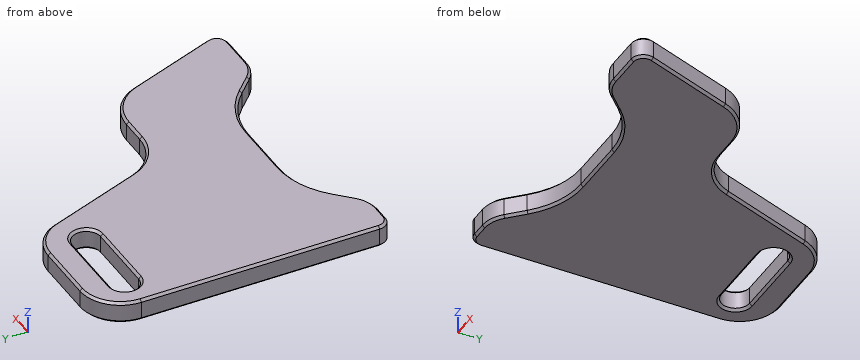
from build123d import *

# Parameters (mm, degrees)
BOSS_EXTRU_1_DEPTH           = 27
ENL_V_MAT_EXTRU_1_DEPTH      = 544.312782602
ENL_V_MAT_EXTRU_1_DEPTH_BACK = 544.312782602
CONG_3_R                     = 60
CONG_4_R                     = 50
CONG_5_R                     = 100
CONG_6_R                     = 15
CONG_7_R                     = 40
ENL_V_MAT_EXTRU_2_DEPTH      = 539.530227365
ENL_V_MAT_EXTRU_2_DEPTH_BACK = 539.530227365
CHANFREIN1_SIZE              = 3


with BuildPart() as part:
    # Esquisse1 → Boss.-Extru.1 (new body)
    with BuildSketch(Plane.XY):
        Polygon((0, 0), (0, 360), (160, 360), (229.154344511, 170), (344.154344511, 170), (406.029284336, 0), align=None)
    extrude(amount=BOSS_EXTRU_1_DEPTH)

    # Esquisse2 → Enlèv. mat.-Extru.1 (cut, two sides: drawn at the far end of the back side and taken through both)
    with BuildSketch(Plane.XY.offset(27).offset(-ENL_V_MAT_EXTRU_1_DEPTH_BACK)):
        Polygon((50, 0), (110, 60), (266.029284336, 60), (326.029284336, 0), align=None)
    extrude(amount=ENL_V_MAT_EXTRU_1_DEPTH + ENL_V_MAT_EXTRU_1_DEPTH_BACK, mode=Mode.SUBTRACT)

    # Congé3
    cong_3_edges = [part.edges().sort_by_distance(p)[0] for p in [
        (229.154344511, 170, 13.5),
        (344.154344511, 170, 13.5),
    ]]
    fillet(cong_3_edges, radius=CONG_3_R)

    # Congé4
    cong_4_edges = [part.edges().sort_by_distance(p)[0] for p in [
        (0, 360, 13.5),
        (160, 360, 13.5),
    ]]
    fillet(cong_4_edges, radius=CONG_4_R)

    # Congé5
    cong_5_edges = [part.edges().sort_by_distance(p)[0] for p in [
        (110, 60, 13.5),
        (266.029284336, 60, 13.5),
    ]]
    fillet(cong_5_edges, radius=CONG_5_R)

    # Congé6
    cong_6_edges = [part.edges().sort_by_distance(p)[0] for p in [
        (0, 0, 13.5),
        (406.029284336, 0, 13.5),
    ]]
    fillet(cong_6_edges, radius=CONG_6_R)

    # Congé7
    cong_7_edges = [part.edges().sort_by_distance(p)[0] for p in [
        (326.029284336, 0, 13.5),
        (50, 0, 13.5),
    ]]
    fillet(cong_7_edges, radius=CONG_7_R)

    # Esquisse3 → Enlèv. mat.-Extru.2 (cut, two sides: drawn at the far end of the back side and taken through both)
    with BuildSketch(Plane.XY.offset(27).offset(-ENL_V_MAT_EXTRU_2_DEPTH_BACK)):
        with BuildLine():
            Line((40, 327.5), (130, 327.5))
            ThreePointArc((130, 327.5), (147.5, 310), (130, 292.5))
            Line((130, 292.5), (40, 292.5))
            ThreePointArc((40, 292.5), (22.5, 310), (40, 327.5))
        make_face()
    extrude(amount=ENL_V_MAT_EXTRU_2_DEPTH + ENL_V_MAT_EXTRU_2_DEPTH_BACK, mode=Mode.SUBTRACT)

    # Chanfrein1
    chanfrein1_edges = [part.edges().sort_by_distance(p)[0] for p in [
        (22.5, 310, 0),
        (85, 327.5, 0),
        (147.5, 310, 0),
        (85, 292.5, 0),
        (22.5, 310, 27),
        (85, 292.5, 27),
        (147.5, 310, 27),
        (85, 327.5, 27),
        (286.654344511, 170, 0),
        (286.654344511, 170, 27),
        (193.379746842, 268.289899283, 0),
        (336.556478399, 159.149122657, 0),
        (193.379746842, 268.289899283, 27),
        (336.556478399, 159.149122657, 27),
        (236.752210622, 180.850877343, 0),
        (236.752210622, 180.850877343, 27),
        (0, 162.5, 0),
        (0, 162.5, 27),
        (87.494811545, 360, 0),
        (153.668444907, 350.957602214, 0),
        (14.644660941, 345.355339059, 0),
        (87.494811545, 360, 27),
        (153.668444907, 350.957602214, 27),
        (14.644660941, 345.355339059, 27),
        (188.014642168, 60, 0),
        (188.014642168, 60, 27),
        (304.8160809, 21.213203436, 27),
        (71.213203436, 21.213203436, 0),
        (262.876271335, 52.387953251, 27),
        (262.876271335, 52.387953251, 0),
        (113.153013001, 52.387953251, 27),
        (113.153013001, 52.387953251, 0),
        (24.215728753, 0, 0),
        (24.215728753, 0, 27),
        (378.612951506, 75.325755375, 0),
        (396.894344899, 6.396353455, 0),
        (4.393398282, 4.393398282, 0),
        (378.612951506, 75.325755375, 27),
        (396.894344899, 6.396353455, 27),
        (4.393398282, 4.393398282, 27),
        (304.8160809, 21.213203436, 0),
        (71.213203436, 21.213203436, 27),
        (363.602445533, 0, 27),
        (48.7387948, 3.0448187, 27),
        (327.290489536, 3.0448187, 27),
        (363.602445533, 0, 0),
        (48.7387948, 3.0448187, 0),
        (327.290489536, 3.0448187, 0),
    ]]
    chamfer(chanfrein1_edges, length=CHANFREIN1_SIZE)


solid = part.part
Verification items for the finished model (mm, model axes). Coordinates: 2 decimals unless noted, no trailing zeros. Order: outer loops, then holes, each group sorted by start corner. A loop starts at its lowest first (then second) coordinate and runs counter-clockwise, first axis right, second up.
Item 1: Depth check by flat-ended pin: pin 1 (4 mm diameter, centred on x = 141, z = 6.5, fed in from +Y); pin 2 (10.5 mm diameter, centred on x = 78, z = 12, fed in from -Y); pin 3 (6.5 mm diameter, centred on x = 194, z = 10, fed in from -Y). Enter the tip coordinate at first touch or a pass-through.
Filled in:
pin 1: stops at y = 358
pin 2: stops at y = 22.75
pin 3: stops at y = 60
Item 2: Section check A-A, the plane z = 15.5. Enter the section's corners in (x, y).
Filled in:
outline: (0, 15) arc R15 ccw to (15, 0) - (33.43, 0) arc R40 ccw to (61.72, 11.72) - (80.71, 30.71) arc R100 cw to (151.42, 60) - (224.61, 60) arc R100 cw to (295.32, 30.71) - (314.31, 11.72) arc R40 ccw to (342.6, 0) - (384.61, 0) arc R15 ccw to (398.7, 20.13) - (358.52, 130.52) arc R60 ccw to (302.14, 170) - (271.17, 170) arc R60 cw to (214.79, 209.48) - (171.97, 327.1) arc R50 ccw to (124.99, 360) - (50, 360) arc R50 ccw to (0, 310) - close; hole (40, 292.5) - (130, 292.5) arc R17.5 ccw to (130, 327.5) - (40, 327.5) arc R17.5 ccw to start
Item 3: Section check C-C, the plane y = 73.5. Enter the section's corners in (x, z), then the cut area to 3 significant figures.
Filled in:
outline: (0, 3) - (3, 0) - (376.08, 0) - (379.28, 3) - (379.28, 24) - (376.08, 27) - (3, 27) - (0, 24) - close
area: 10,200 mm2
Item 4: Section check B-B, the plane x = 206. Enter the section's corners in (y, z), then the cut area to 3 significant figures.
Filled in:
outline: (60, 3) - (63, 0) - (224.84, 0) - (233.62, 3) - (233.62, 24) - (224.84, 27) - (63, 27) - (60, 24) - close
area: 4,650 mm2
Item 5: Material ranges on L1, parallel to X at y = 312.5, z = 15.5; L2, parallel to X at y = 302, z = 15; L3, parallel to Y at x = 121, z = 23.75, recorded low to high.
Filled in:
L1: x = 0.06 to 22.68, 147.32 to 177.29
L2: x = 0 to 24.44, 145.56 to 181.11
L3: y = 55.26 to 292.5, 327.5 to 360
